Geometry: see drawing. Coordinates: mm, zero at the bounding-box minimum. A direction names the side the tool comes from. Give positions to 0.01 mm unless a question says otherwise; leave off trailing zeros. Order: outer loops, then holes, each group sorted by start corner. A loop starts at its lowest first (then second) coordinate and runs counter-clockwise, first axis right, second up. Notation, with made-up numbers: (85, 84) - (118, 84) arc R14 ccw to (118, 96) - close; hole circle Ø2 at (16, 64.5). An arc over 180 degrees is marked (long way). One line per item, written item: value.
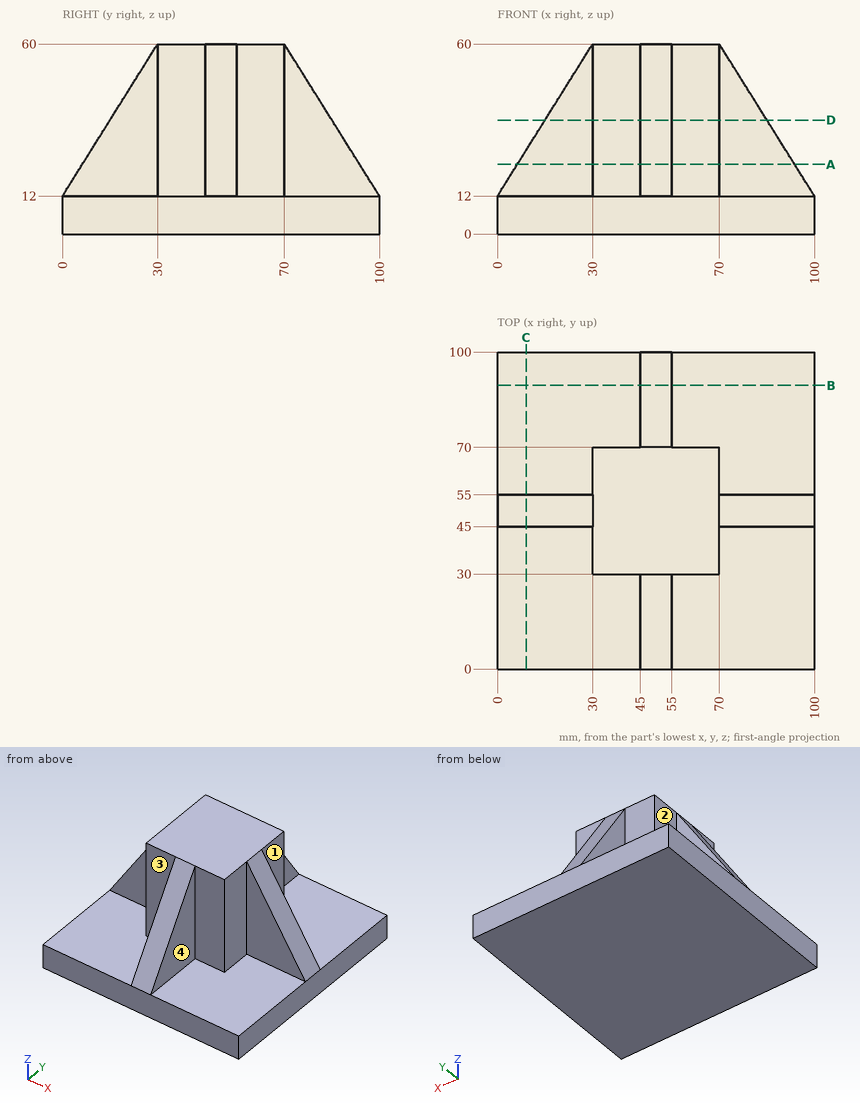
1) Section D-D, the plane z = 36. Return loops of the section in (x, y), then the cut area to 3 significant figures.
Answers below:
outline: (15, 45) - (30, 45) - (30, 30) - (45, 30) - (45, 15) - (55, 15) - (55, 30) - (70, 30) - (70, 45) - (85, 45) - (85, 55) - (70, 55) - (70, 70) - (55, 70) - (55, 85) - (45, 85) - (45, 70) - (30, 70) - (30, 55) - (15, 55) - close
area: 2,200 mm^2
2) First-contact query: pin 1 (1.5 mm diameter, centred on x = 69.5, z = 39, fed in from +Y); pin 2 (15 mm diameter, centred on x = 10.5, z = 32.5, fed in from -Y); pin 3 (24 mm diameter, centred on y = 21, z = 44, fed in from -X). Flat tips, straight axial feed; report the tip coordinate or a pass-through.
Answers below:
pin 1: y = 70
pin 2: y = 45
pin 3: x = 30
3) Section C-C, the plane x = 9. Return loops of the section in (y, z), then the cut area to 3 significant figures.
Answers below:
outline: (0, 0) - (100, 0) - (100, 12) - (55, 12) - (55, 26.4) - (45, 26.4) - (45, 12) - (0, 12) - close
area: 1,340 mm^2
4) Material intervals for line 1 along X through (y, z) = (94.5, 17); line 2 along Z through (x, y) = (37, 4); line 3 along Y through (x, z) = (40.5, 29), sorted ascending.
Answers below:
line 1: 45 to 55
line 2: 0 to 12
line 3: 30 to 70
5) Section B-B, the plane y = 89.5. Return loops of the section in (x, z).
Answers below:
outline: (0, 0) - (100, 0) - (100, 12) - (55, 12) - (55, 28.8) - (45, 28.8) - (45, 12) - (0, 12) - close
6) Section A-A, the plane z = 22. Return loops of the section in (x, y).
Answers below:
outline: (6.25, 45) - (30, 45) - (30, 30) - (45, 30) - (45, 6.25) - (55, 6.25) - (55, 30) - (70, 30) - (70, 45) - (93.75, 45) - (93.75, 55) - (70, 55) - (70, 70) - (55, 70) - (55, 93.75) - (45, 93.75) - (45, 70) - (30, 70) - (30, 55) - (6.25, 55) - close
7) Set-up query: the marked faces 1, 2, 3 and 4. Return all of +Z, -Z, +X, -X, +Y, -Y with unobstructed straight access to the full face (end or side cutting, diameter ignored); none if empty.
Answers below:
face 1: +Z, +X, +Y
face 2: +Z, -X, +Y
face 3: +Z, -X, -Y
face 4: +Z, +X, -Y
